Source: three-view drawing plus pictorial views. Frame: mm from the lowest corner of the part. Coordinates: 2 decimals unless noted, no trailing zeros. Loops run counter-clockwise (first coordinate to the right, second up) from the corner with the lowest first, then second, coordinate; pieces in that order, holes last. Notation, with made-up numbers: (64.25, -30.5) - (68.25, -30.5) arc R19 ccw to (68.25, -20.5) - close; hole circle Ø1 at (18, 66.25). An arc over 180 degrees is marked (long way). Return JSON: item names as keys, results as strings.
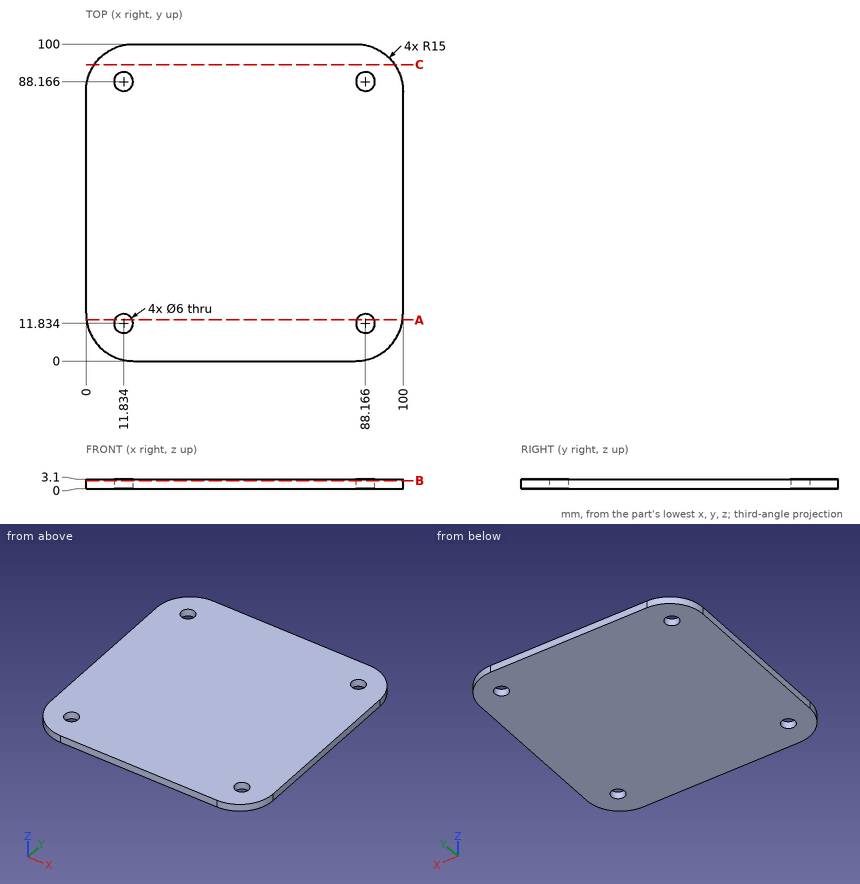
Item 1: Section query A-A, the plane y = 13. Return loops of the section in (x, z).
Worked out:
{"outline": "(0.13, 0) - (9.07, 0) - (9.07, 3.1) - (0.13, 3.1) - close; (14.6, 0) - (85.4, 0) - (85.4, 3.1) - (14.6, 3.1) - close; (90.93, 0) - (99.87, 0) - (99.87, 3.1) - (90.93, 3.1) - close"}
Item 2: Section query C-C, the plane y = 93.5. Return loops of the section in (x, z).
Worked out:
{"outline": "(2.64, 0) - (97.36, 0) - (97.36, 3.1) - (2.64, 3.1) - close"}
Item 3: Section query B-B, the plane z = 2.6. Return loops of the section in (x, y).
Worked out:
{"outline": "(0, 15) arc R15 ccw to (15, 0) - (85, 0) arc R15 ccw to (100, 15) - (100, 85) arc R15 ccw to (85, 100) - (15, 100) arc R15 ccw to (0, 85) - close; hole circle Ø6 at (11.83, 11.83); hole circle Ø6 at (11.83, 88.17); hole circle Ø6 at (88.17, 11.83); hole circle Ø6 at (88.17, 88.17)"}
Item 4: Ray query, probe 1 along X at (y, z) = (90.5, 0.4) (1 decimal); probe 2 along Y at (x, z) = (85.5, 1.95); probe 3 along X at (y, z) = (87.5, 0.45). Return the intervals inside material, ascending. Write a range as from..to.
Worked out:
{"probe 1": "1..9.9, 13.7..86.3, 90.1..99", "probe 2": "0.01..10.46, 13.21..86.79, 89.54..99.99", "probe 3": "0.21..8.91, 14.76..85.24, 91.09..99.79"}
